Design review of the part shown in the three views and the two pictorial views. Dimensions are in mm from the part's minimum x, y and z. Give positions to 0.01 mm unless a question says otherwise; leave off trailing zeros. Loops run counter-clockwise (first coordinate to the right, second up) from the corner with the lowest first, then second, coordinate; pieces in that order, holes last. Notation, with made-up numbers: (-16, -10) - (41, -10) arc R15 cw to (41, 10) - close; hole circle Ø2 at (51, -18.5). An arc over 180 degrees is marked (long way). Return JSON: item names as keys, results as strings. Group by question number.
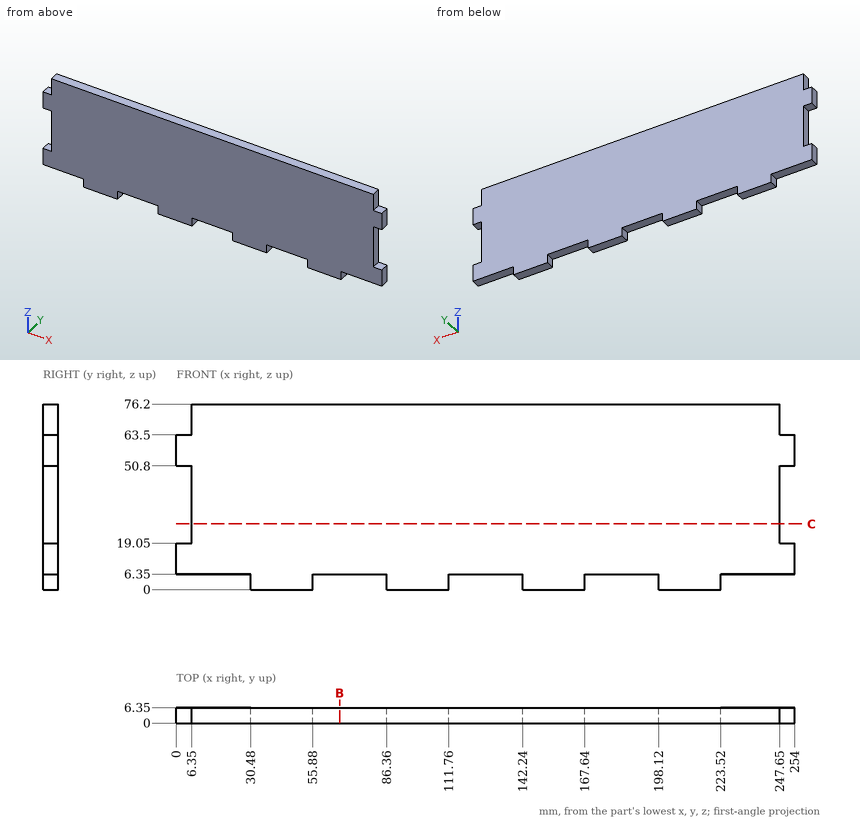
Item 1: For P1, Ø1.9, axis at y = 3.5, z = 4, coming from the +X side; P2, Ø2, axis at x = 202, z = 23, coming from the -Y side; P3, Ø1.9, axis at y = 3, z = 67, coming from the +X side; P4, Ø3, axis at y = 3.5, z = 2.5, coming from the -X side, all flat-tipped, find the tip position at first contact; note any pin that passes through.
Item 2: Take a section at C-C (z = 27). State the section outline as (x, y) points, then the cut area to 3 significant figures.
Item 3: For L1, parallel to X at y = 5.5, z = 6; L2, parallel to Z at x = 129, y = 4.5; L3, parallel to X at y = 0.5, z = 20, list the stretches that pass through material, from the lowest coordinate up. Write a range as from..to.
Item 4: Take a section at B-B (x = 67). State the section outline as (y, z) points, then the cut area to 3 significant figures.
Check sheet entries:
{
 "1": {"P1": "stops at x = 223.52", "P2": "stops at y = 0", "P3": "stops at x = 247.65", "P4": "stops at x = 30.48"},
 "2": {"outline": "(6.35, 0) - (247.65, 0) - (247.65, 6.35) - (6.35, 6.35) - close", "area": "1,530 mm^2"},
 "3": {"L1": "x = 30.48..55.88, 86.36..111.76, 142.24..167.64, 198.12..223.52", "L2": "z = 6.35..76.2", "L3": "x = 6.35..247.65"},
 "4": {"outline": "(0, 6.35) - (6.35, 6.35) - (6.35, 76.2) - (0, 76.2) - close", "area": "444 mm^2"}
}
